Geometry check sheet. Reference: drawing and pictorial views, mm from the part's lowest x, y, z. Round coordinates to 2 decimals unless told otherwise and drop trailing zeros. Write each loop counter-clockwise with the first axis right and the second up, starting at its lowest first coordinate (ties: lowest second). Pieces come first, ordered by that corner, then holes. Notation, with made-up numbers: M -0.5,-33.5 L 54.5,-33.5 A26 cw 54.5,-14.5 Z; hole C 7,13 d6. An arc over 180 degrees is marked long. Put each result on its own line as item: value. Start each with the question number.
(1) Section check C-C on y = 10. Record the cut outline in (x, z), then the cut area to 3 significant figures.
(2) Section check A-A on z = 28.5. Record the cut outline in (x, y).
(3) Section check B-B on x = 2.5. Record the cut outline in (y, z) (1 decimal), then the cut area to 4 significant figures.
(4) Gauge pin test, flat ends, axial feed: pin 1 (4.5 mm diameter, centred on x = 6.4, y = 6.4, fed in from +Z); pin 2 (6 mm diameter, centred on y = 3, z = 42, fed in from +X); pin 3 (1 mm diameter, centred on x = 4, z = 41, fed in from +Y); pin 4 (6 mm diameter, centred on x = 10.5, z = 40, fed in from +Y) (1 decimal). Record the tip position at first contact, or that the pin passes through.
(5) Material ranges on probe 1 along Y at (x, z) = (6.4, 3); probe 2 along X at (y, z) = (6.75, 59.5), recorded low to high.
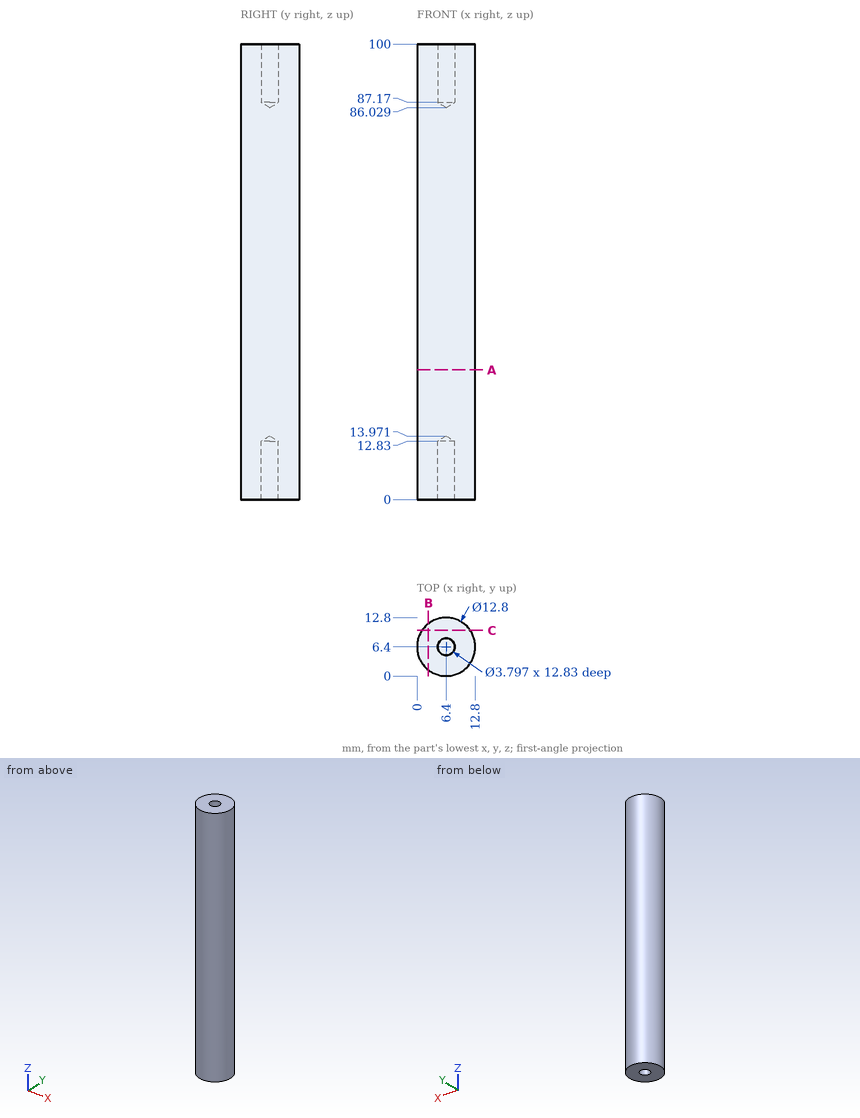
Answers follow:
1. outline: M 1.11,0 L 11.69,0 L 11.69,100 L 1.11,100 Z
1. area: 1,060 mm^2
2. outline: C 6.4,6.4 d12.8
3. outline: M 1.3,0 L 11.5,0 L 11.5,100 L 1.3,100 Z
3. area: 1,015 mm^2
4. pin 1: stops at z = 100
4. pin 2: stops at x = 12.79
4. pin 3: stops at y = 12.51
4. pin 4: stops at y = 12.7
5. probe 1: y = 0 to 4.5, 8.3 to 12.8
5. probe 2: x = 0.01 to 12.79
